Here's how the part is built. I have some questions about the finished solid (model axes, mm). A direction names the side the tool comes from. Round coordinates to 2 decimals unless told otherwise and drop trailing zeros. Order: outer loops, then holes, each group sorted by start corner. A loop starts at its lowest first (then second) coordinate and runs counter-clockwise, first axis right, second up. Notation, with made-up numbers: M 73.25,9 L 89.25,9 A31 cw 89.25,45 Z; hole C -35,-24 d5. An arc over 180 degrees is marked long. Use one line per item in the form item = value. Start each with the question number.
```python
from build123d import *

# Parameters (mm, degrees)
SKETCH1_R               = 2.54
BOSS_EXTRUDE1_DEPTH     = 11.43
SKETCH2_R               = 1.27
BOSS_EXTRUDE2_DEPTH     = 1.27
CUT_EXTRUDE1_DEPTH      = 14.198227154
CUT_EXTRUDE1_DEPTH_BACK = 14.198227154
SKETCH3_R               = 0.381
SCALE1_SCALE            = 1.5


with BuildPart() as part:
    # Sketch1 → Boss-Extrude1 (new body)
    with BuildSketch(Plane(origin=(0, 0, 0), x_dir=(1, 0, 0), z_dir=(0, 1, 0))):
        with Locations(Location((0, 0, 0), (0, 0, 270))):
            Circle(SKETCH1_R)
    extrude(amount=BOSS_EXTRUDE1_DEPTH)

    # Sketch2 → Boss-Extrude2 (add)
    with BuildSketch(Plane(origin=(0, 11.43, 0), x_dir=(1, 0, 0), z_dir=(0, 1, 0))):
        with Locations(Location((0, 0, 0), (0, 0, 270))):
            Circle(SKETCH2_R)
    extrude(amount=BOSS_EXTRUDE2_DEPTH)

    # Sketch3 → Cut-Extrude1 (cut, two sides: drawn at the far end of the back side and taken through both)
    with BuildSketch(Plane(origin=(0, 0, 0), x_dir=(0, 0, -1), z_dir=(1, 0, 0)).offset(-CUT_EXTRUDE1_DEPTH_BACK)):
        with Locations((0, 12.065)):
            Circle(SKETCH3_R)
    extrude(amount=CUT_EXTRUDE1_DEPTH + CUT_EXTRUDE1_DEPTH_BACK, mode=Mode.SUBTRACT)


with BuildPart() as part_1:
    # Scale1: scaled about (0, 5.856765052, -1.11e-07)
    add(part.part.scale(SCALE1_SCALE).moved(Location((0, -2.928382526, 5.6e-08))))


solid = part_1.part
```
1) If we section it at C-C on y = -0.5: Write out the boundary of the cut face in (x, z), then the cut area to 3 significant figures.
2) If we mould it in two halves opening along Z, with no side actions, what happens to faces 3 (the flat face through (0, 16.122, 0)), 4 (the cylindrical face through (-0.027, 15.736, 0.074)), 5 (the cylindrical face through (-1.69, 15.16, 0.88))? For each: +Z half, -Z half, draft (parallel to the pull), parting line (faces both ways), or undercut.
3) If we section it at A-A on z = 0: Write out the boundary of the cut face in (x, y) (3 decimals), then the cut area to 3 significant figures.
4) On a 3-axis mill with a long thin cutter (end or side, diameter ignored), from which of +Z, -Z, +X, -X, +Y, -Y can I reach the whole of each face in a straight line? I mean faces 1 (the flat face through (0, -2.928, 0)), 2 (the flat face through (2, 14.217, 1)). Say none if no direction works.
5) Will these pins go through, and if not, where does the flat tip stop? pin 1 Ø1 at (x, z) = (1, -2) entering from +Y; pin 2 Ø2 at (y, z) = (5, -2) entering from -X; pin 3 Ø1.3 at (y, z) = (15.17, 0) entering from +X (3 decimals); pin 4 Ø1 at (y, z) = (7, 1.5) entering from +X.
6) If we section it at B-B on x = 0: Write out the boundary of the cut face in (y, z) (1 decimal).
7) If I drill on line 1 (Y direction, x = 1.15, z = 0); line 2 (Y direction, x = 0.75, z = 2); line 3 (Y direction, x = -0.75, z = 0.25), over which ranges is the centre line in solid material (lowest first)?
8) If we section it at D-D on z = -1: Write out the boundary of the cut face in (x, y), then the cut area to 3 significant figures.
Completed:
q1.outline = C 0,0 d7.62
q1.area = 45.6 mm²
q2.face_3 = draft
q2.face_4 = undercut
q2.face_5 = parting line
q3.outline = M -3.81,-2.928 L 3.81,-2.928 L 3.81,14.217 L 1.905,14.217 L 1.905,14.598 L -1.905,14.598 L -1.905,14.217 L -3.81,14.217 Z; M -1.905,15.741 L 1.905,15.741 L 1.905,16.122 L -1.905,16.122 Z
q3.area = 134 mm²
q4.face_1 = +Z, -Z, +X, -X, -Y
q4.face_2 = +Y
q5.pin_1 = 16.12
q5.pin_2 = -3.68
q5.pin_3 = 1.905
q5.pin_4 = 3.68
q6.outline = M -2.9,-3.8 L 14.2,-3.8 L 14.2,-1.9 L 16.1,-1.9 L 16.1,1.9 L 14.2,1.9 L 14.2,3.8 L -2.9,3.8 Z; hole C 15.2,0 d1.1
q7.line_1 = -2.93 to 14.6, 15.74 to 16.12
q7.line_2 = -2.93 to 14.22
q7.line_3 = -2.93 to 14.66, 15.68 to 16.12
q8.outline = M -3.68,-2.93 L 3.68,-2.93 L 3.68,14.22 L 1.62,14.22 L 1.62,16.12 L -1.62,16.12 L -1.62,14.22 L -3.68,14.22 Z
q8.area = 132 mm²
